Check sheet for the modelled part. Datum: model origin and axes. Units: mm. A direction names the side the tool comes from. Round coordinates to 2 decimals unless told otherwise and drop trailing zeros. Write each loop counter-clockwise with the first axis right and the second up, starting at its lowest first coordinate (ties: lowest second). Pieces come first, ordered by that corner, then holes. Notation, with made-up numbers: M 13.25,71.5 L 63.25,71.5 A25 ccw 63.25,86.5 Z; hole C 71.25,20.25 d10. An arc over 180 degrees is marked long. One line per item, written item: value.
from build123d import *

# Parameters (mm, degrees)
EXTRUDE_1_DEPTH = 2.2
EXTRUDE_2_DEPTH = 2.2
FILLET_1_R      = 2


with BuildPart() as part:
    # 草图1 → 凸台-拉伸1 (new body)
    with BuildSketch(Plane(origin=(0, 0, 0), x_dir=(0, 0, -1), z_dir=(1, 0, 0))):
        with BuildLine():
            Line((-20.1, -17.25), (20.1, -17.25))
            Line((20.1, -17.25), (20.1, -1.311067127))
            Line((20.1, -1.311067127), (28, 3.25))
            Line((28, 3.25), (28, 5.24))
            ThreePointArc((28, 5.24), (26.995, 6.245), (28, 7.25))
            Line((28, 7.25), (31, 7.25))
            Line((31, 7.25), (31, 13.25))
            Line((31, 13.25), (28, 13.25))
            ThreePointArc((28, 13.25), (26.995, 14.255), (28, 15.26))
            Line((28, 15.26), (28, 17.25))
            Line((28, 17.25), (10.9, 17.25))
            Line((10.9, 17.25), (10.9, -7.25))
            Line((10.9, -7.25), (-10.9, -7.25))
            Line((-10.9, -7.25), (-10.9, 17.25))
            Line((-10.9, 17.25), (-28, 17.25))
            Line((-28, 17.25), (-28, 15.26))
            ThreePointArc((-28, 15.26), (-27.289357685, 14.965642315), (-26.995, 14.255))
            ThreePointArc((-26.995, 14.255), (-27.289357685, 13.544357685), (-28, 13.25))
            Line((-28, 13.25), (-31, 13.25))
            Line((-31, 13.25), (-31, 7.25))
            Line((-31, 7.25), (-28, 7.25))
            ThreePointArc((-28, 7.25), (-27.289357685, 6.955642315), (-26.995, 6.245))
            ThreePointArc((-26.995, 6.245), (-27.289357685, 5.534357685), (-28, 5.24))
            Line((-28, 5.24), (-28, 3.25))
            Line((-28, 3.25), (-20.1, -1.311067127))
            Line((-20.1, -1.311067127), (-20.1, -17.25))
        make_face()
        with BuildLine():
            Line((-7.91, -14.4), (-14.09, -14.4))
            ThreePointArc((-14.09, -14.4), (-15.095, -15.405), (-16.1, -14.4))
            Line((-16.1, -14.4), (-16.1, -12.1))
            ThreePointArc((-16.1, -12.1), (-15.095, -11.095), (-14.09, -12.1))
            Line((-14.09, -12.1), (-7.91, -12.1))
            ThreePointArc((-7.91, -12.1), (-6.905, -11.095), (-5.9, -12.1))
            Line((-5.9, -12.1), (-5.9, -14.4))
            ThreePointArc((-5.9, -14.4), (-6.905, -15.405), (-7.91, -14.4))
        make_face(mode=Mode.SUBTRACT)
        with BuildLine():
            Line((16.1, -12.1), (16.1, -14.4))
            ThreePointArc((16.1, -14.4), (15.095, -15.405), (14.09, -14.4))
            Line((14.09, -14.4), (7.91, -14.4))
            ThreePointArc((7.91, -14.4), (6.905, -15.405), (5.9, -14.4))
            Line((5.9, -14.4), (5.9, -12.1))
            ThreePointArc((5.9, -12.1), (6.905, -11.095), (7.91, -12.1))
            Line((7.91, -12.1), (14.09, -12.1))
            ThreePointArc((14.09, -12.1), (15.095, -11.095), (16.1, -12.1))
        make_face(mode=Mode.SUBTRACT)
        with BuildLine():
            Line((-15.91, 12.1), (-22.09, 12.1))
            ThreePointArc((-22.09, 12.1), (-23.095, 11.095), (-24.1, 12.1))
            Line((-24.1, 12.1), (-24.1, 14.4))
            ThreePointArc((-24.1, 14.4), (-23.095, 15.405), (-22.09, 14.4))
            Line((-22.09, 14.4), (-15.91, 14.4))
            ThreePointArc((-15.91, 14.4), (-14.905, 15.405), (-13.9, 14.4))
            Line((-13.9, 14.4), (-13.9, 12.1))
            ThreePointArc((-13.9, 12.1), (-14.905, 11.095), (-15.91, 12.1))
        make_face(mode=Mode.SUBTRACT)
        with BuildLine():
            Line((13.9, 12.1), (13.9, 14.4))
            ThreePointArc((13.9, 14.4), (14.905, 15.405), (15.91, 14.4))
            Line((15.91, 14.4), (22.09, 14.4))
            ThreePointArc((22.09, 14.4), (23.095, 15.405), (24.1, 14.4))
            Line((24.1, 14.4), (24.1, 12.1))
            ThreePointArc((24.1, 12.1), (23.095, 11.095), (22.09, 12.1))
            Line((22.09, 12.1), (15.91, 12.1))
            ThreePointArc((15.91, 12.1), (14.905, 11.095), (13.9, 12.1))
        make_face(mode=Mode.SUBTRACT)
    extrude(amount=EXTRUDE_1_DEPTH)

    # 草图2 → 凸台-拉伸2 (add)
    with BuildSketch(Plane(origin=(2.2, 0, 0), x_dir=(0, 0, -1), z_dir=(1, 0, 0))):
        Polygon((-11.5, -17.25), (-11.5, -22.25), (11.5, -22.25), (11.5, -17.25), (7.5, -17.25), (7.5, -19.26), (-7.5, -19.26), (-7.5, -17.25), align=None)
    extrude(amount=-EXTRUDE_2_DEPTH)

    # 圆角1
    # the kernel refuses this fillet: 2 mm, written as the material it adds along each edge
    with BuildSketch(Plane(origin=(0, -1.311067127, -20.1), x_dir=(0, -1, 0), z_dir=(1, 0, 0)), Plane(origin=(0, -1.311067127, 20.1), x_dir=(0, 0.49999999999999634, 0.8660254037844408), z_dir=(1, 0, 0))) as fillet_1_piece_1:
        with BuildLine():
            CenterArc((FILLET_1_R * 0.57735026919, FILLET_1_R), FILLET_1_R, 210, 60)
            Line((-FILLET_1_R * 0.288675134595, FILLET_1_R * 0.5), (0, 0))
            Line((0, 0), (FILLET_1_R * 0.57735026919, 0))
        make_face()
    extrude(amount=2.2)
    with BuildSketch(Plane(origin=(0, -7.25, -10.9), x_dir=(0, 1, 0), z_dir=(1, 0, 0)), Plane(origin=(0, -7.25, 10.9), x_dir=(0, 0, -1), z_dir=(1, 0, 0)), Plane(origin=(2.2, -17.25, 7.5), x_dir=(0, 0, -1), z_dir=(-1, 0, 0)), Plane(origin=(2.2, -17.25, -11.5), x_dir=(0, 0, -1), z_dir=(-1, 0, 0))) as fillet_1_piece_2:
        with BuildLine():
            CenterArc((FILLET_1_R, FILLET_1_R), FILLET_1_R, 180, 90)
            Line((0, FILLET_1_R), (0, 0))
            Line((0, 0), (FILLET_1_R, 0))
        make_face()
    extrude(amount=2.2)
    with BuildSketch(Plane(origin=(2.2, -19.26, -7.5), x_dir=(0, 1, 0), z_dir=(-1, 0, 0)), Plane(origin=(2.2, -19.26, 7.5), x_dir=(0, 0, -1), z_dir=(-1, 0, 0)), Plane(origin=(2.2, -17.25, -7.5), x_dir=(0, 0, 1), z_dir=(-1, 0, 0)), Plane(origin=(2.2, -17.25, 11.5), x_dir=(0, 0, 1), z_dir=(-1, 0, 0))) as fillet_1_piece_3:
        with BuildLine():
            CenterArc((FILLET_1_R, -FILLET_1_R), FILLET_1_R, 90, 90)
            Line((0, -FILLET_1_R), (0, 0))
            Line((0, 0), (FILLET_1_R, 0))
        make_face()
    extrude(amount=2.2)
    # the kernel refuses this fillet: 2 mm, written as the material it takes off along each edge
    with BuildSketch(Plane(origin=(-5, -17.25, 20.1), x_dir=(0, 1, 0), z_dir=(1, 0, 0)), Plane(origin=(-5, -17.25, -20.1), x_dir=(0, 0, 1), z_dir=(1, 0, 0)), Plane(origin=(-5, 17.25, -10.9), x_dir=(0, 0, -1), z_dir=(1, 0, 0)), Plane(origin=(-5, 17.25, 10.9), x_dir=(0, -1, 0), z_dir=(1, 0, 0))) as fillet_1_2_piece_1:
        with BuildLine():
            CenterArc((FILLET_1_R, -FILLET_1_R), FILLET_1_R, 90, 90)
            Line((0, -FILLET_1_R), (0, 0))
            Line((0, 0), (FILLET_1_R, 0))
        make_face()
    extrude(amount=12.2, mode=Mode.SUBTRACT)
    with BuildSketch(Plane(origin=(7.2, -22.25, -11.5), x_dir=(0, 0, 1), z_dir=(-1, 0, 0)), Plane(origin=(7.2, -22.25, 11.5), x_dir=(0, 1, 0), z_dir=(-1, 0, 0))) as fillet_1_2_piece_2:
        with BuildLine():
            CenterArc((FILLET_1_R, FILLET_1_R), FILLET_1_R, 180, 90)
            Line((0, FILLET_1_R), (0, 0))
            Line((0, 0), (FILLET_1_R, 0))
        make_face()
    extrude(amount=12.2, mode=Mode.SUBTRACT)


solid = part.part
Q1. Access from +Z, -Z, +X, -X, +Y, -Y to the whole of each face (thin tool, end or side, straight path). Record for faces 1 (the cylindrical face through (1.08, 16.65, 11.47)), 2 (the flat face through (1, -17.25, 16)), 3 (the cylindrical face through (1.12, -17.51, -6.49)), 4 (the flat face through (1, 4, -28)).
Completed:
face 1: +X, -X, +Y
face 2: +Z, +X, -X, -Y
face 3: +X, -X
face 4: -Z, +X, -X, -Y
Q2. Sectioned sample at A-A on z = -0.5. Enter the section's corners in (x, y).
Completed:
outline: M 0,-22.25 L 2.2,-22.25 L 2.2,-19.26 L 0,-19.26 Z; M 0,-17.25 L 2.2,-17.25 L 2.2,-7.25 L 0,-7.25 Z
Q3. Sectioned sample at B-B on y = 9. Enter the section's corners in (x, z), and give its area (3 significant figures).
Completed:
outline: M 0,-31 L 2.2,-31 L 2.2,-10.9 L 0,-10.9 Z; M 0,10.9 L 2.2,10.9 L 2.2,31 L 0,31 Z
area: 88.4 mm^2
Q4. Sectioned sample at C-C on y = -13.5. Enter the section's corners in (x, z).
Completed:
outline: M 0,-20.1 L 2.2,-20.1 L 2.2,-16.1 L 0,-16.1 Z; M 0,-5.9 L 2.2,-5.9 L 2.2,5.9 L 0,5.9 Z; M 0,16.1 L 2.2,16.1 L 2.2,20.1 L 0,20.1 Z
Q5. Depth check by flat-ended pin: P1, Ø1.1, axis at x = 1, z = -29, coming from the +Y side; P2, Ø1.1, axis at x = 0.5, y = -11.5, coming from the -Z side; P3, Ø0.6, axis at x = 0.5, y = 16, coming from the -Z side. Enter the tip coordinate at first touch or a pass-through.
Completed:
P1: y = 13.25
P2: z = -20.1
P3: z = -28
Q6. Draft check along Z on faces 5 (the flat face through (1, 10, -31)), 6 (the cylindrical face through (1.08, -16.65, 19.53)), 7 (the flat face through (0, -11, 0)), 8 (the cylindrical face through (1.085, -11.095, 15.117)). Enter one of: pulls with the +Z half, pulls with the -Z half, needs draft (parallel to the pull), parting line crosses it, or undercut.
Completed:
face 5: pulls with the -Z half
face 6: pulls with the +Z half
face 7: needs draft
face 8: undercut
Q7. Scan lines: line 1 (Z direction, x = 0.95, y = -12); line 2 (Z direction, x = 0.95, y = -14); line 3 (Z direction, x = 0.55, y = 9). Record each from-to range of solid material in increasing order. Write a range as [from, to].
Completed:
line 1: [-20.1, -16.1], [-14.09, -7.91], [-5.9, 5.9], [7.91, 14.09], [16.1, 20.1]
line 2: [-20.1, -16.1], [-5.9, 5.9], [16.1, 20.1]
line 3: [-31, -10.9], [10.9, 31]
Q8. Sectioned sample at D-D on x = 0.7. State how many separate pieces and enclosed holes the cut face has, and give its area (3 significant figures).
Completed:
separate pieces: 1
enclosed holes: 5
area: 1,110 mm^2
